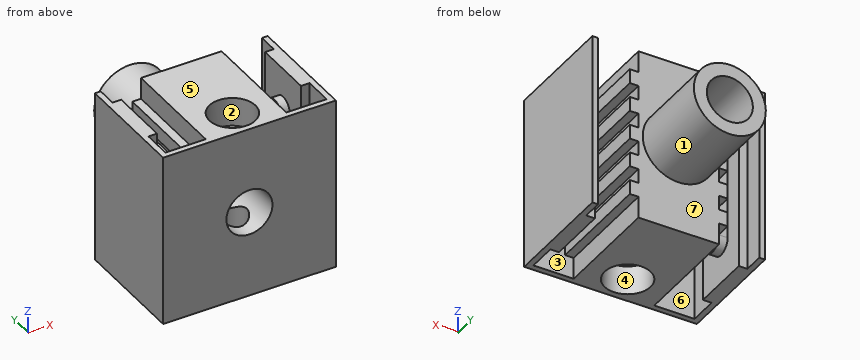
```python
from build123d import *

# Parameters (mm, degrees)
ESBO_O1_R                = 12.5
RESSALTO_EXTRUS_O1_DEPTH = 30
ESBO_O2_R                = 8
CORTE_EXTRUS_O1_DEPTH    = 15
ESBO_O3_W                = 3
ESBO_O3_H                = 5
CORTE_EXTRUS_O2_DEPTH    = 6.5
ESBO_O4_W                = 60
ESBO_O4_H                = 60
RESSALTO_EXTRUS_O2_DEPTH = 40
ESBO_O5_W                = 11
ESBO_O5_H                = 60
CORTE_EXTRUS_O3_DEPTH    = 35
ESBO_O6_W                = 11
ESBO_O6_H                = 60
CORTE_EXTRUS_O4_DEPTH    = 38
ESBO_O7_W                = 60
ESBO_O7_H                = 21
RESSALTO_EXTRUS_O3_DEPTH = 3.00002654
ESBO_O8_W                = 60
ESBO_O8_H                = 21
RESSALTO_EXTRUS_O4_DEPTH = 3.004451555
RESSALTO_EXTRUS_O5_DEPTH = 2.995218695
RESSALTO_EXTRUS_O6_START = 3
RESSALTO_EXTRUS_O6_DEPTH = 3
ESBO_O15_R               = 8
CORTE_EXTRUS_O5_DEPTH    = 70.462219947
ESBO_O19_W               = 5
ESBO_O19_H               = 38
ESBO_O19_W_2             = 7.5
CORTE_EXTRUS_O7_DEPTH    = 3
ESBO_O20_W               = 7.5
ESBO_O20_H               = 38
ESBO_O20_W_2             = 5
CORTE_EXTRUS_O8_DEPTH    = 3
ESBO_O21_R               = 8
CORTE_EXTRUS_O9_DEPTH    = 10
CORTE_EXTRUS_O10_START   = -10
ESBO_O22_R               = 8
CORTE_EXTRUS_O10_DEPTH   = 10
ESBO_O24_R               = 5
CORTE_EXTRUS_O11_DEPTH   = 71.710678119


with BuildPart() as part:
    # Esboço1 → Ressalto-extrusão1 (new body)
    with BuildSketch(Plane(origin=(0, 0, 0), x_dir=(1, 0, 0), z_dir=(0, 1, 0))):
        with Locations(Location((0, 0, 0), (0, 0, 270))):
            Circle(ESBO_O1_R)
    extrude(amount=RESSALTO_EXTRUS_O1_DEPTH)

    # Esboço2 → Corte-extrusão1 (cut)
    with BuildSketch(Plane(origin=(0, 30, 0), x_dir=(1, 0, 0), z_dir=(0, 1, 0))):
        with Locations(Location((0, 0, 0), (0, 0, 270))):
            Circle(ESBO_O2_R)
    extrude(amount=-CORTE_EXTRUS_O1_DEPTH, mode=Mode.SUBTRACT)

    # Esboço3 → Corte-extrusão2 (cut)
    with BuildSketch(Plane.XZ):
        Rectangle(ESBO_O3_W, ESBO_O3_H)
    extrude(amount=-CORTE_EXTRUS_O2_DEPTH, mode=Mode.SUBTRACT)

    # Esboço4 → Ressalto-extrusão2 (add)
    with BuildSketch(Plane.XZ):
        Rectangle(ESBO_O4_W, ESBO_O4_H)
    extrude(amount=RESSALTO_EXTRUS_O2_DEPTH)

    # Esboço5 → Corte-extrusão3 (cut)
    with BuildSketch(Plane(origin=(0, 0, 0), x_dir=(1, 0, 0), z_dir=(0, 1, 0))):
        with Locations((-22.5, 0)):
            Rectangle(ESBO_O5_W, ESBO_O5_H)
        with Locations((22.5, 0)):
            Rectangle(ESBO_O5_W, ESBO_O5_H)
    extrude(amount=-CORTE_EXTRUS_O3_DEPTH, mode=Mode.SUBTRACT)

    # Esboço6 → Corte-extrusão4 (cut)
    with BuildSketch(Plane(origin=(0, 0, 0), x_dir=(1, 0, 0), z_dir=(0, 1, 0))):
        with Locations((-22.5, 0)):
            Rectangle(ESBO_O6_W, ESBO_O6_H)
        with Locations((22.5, 0)):
            Rectangle(ESBO_O6_W, ESBO_O6_H)
    extrude(amount=-CORTE_EXTRUS_O4_DEPTH, mode=Mode.SUBTRACT)

    # Esboço7 → Ressalto-extrusão3 (add)
    with BuildSketch(Plane(origin=(-28, 0, 0), x_dir=(0, 0, -1), z_dir=(1, 0, 0))):
        with Locations((0, -17.5)):
            Rectangle(ESBO_O7_W, ESBO_O7_H)
    extrude(amount=RESSALTO_EXTRUS_O3_DEPTH)

    # Esboço8 → Ressalto-extrusão4 (add)
    with BuildSketch(Plane.ZY.offset(-28)):
        with Locations((0, -17.5)):
            Rectangle(ESBO_O8_W, ESBO_O8_H)
    extrude(amount=RESSALTO_EXTRUS_O4_DEPTH)

    # Esboço9 → Ressalto-extrusão5 (add)
    with BuildSketch(Plane.ZY.offset(-24.995548445)):
        with BuildLine():
            Line((-16, -13.5), (16, -13.5))
            ThreePointArc((16, -13.5), (20, -17.5), (16, -21.5))
            Line((16, -21.5), (-16, -21.5))
            ThreePointArc((-16, -21.5), (-20, -17.5), (-16, -13.5))
        make_face()
    extrude(amount=RESSALTO_EXTRUS_O5_DEPTH)

    # Esboço14 → Ressalto-extrusão6 (add)
    with BuildSketch(Plane(origin=(-24.99997346, 0, 0), x_dir=(0, 0, -1), z_dir=(1, 0, 0)).offset(RESSALTO_EXTRUS_O6_START)):
        with BuildLine():
            Line((-16, -13.5), (16, -13.5))
            ThreePointArc((16, -13.5), (20, -17.5), (16, -21.5))
            Line((16, -21.5), (-16, -21.5))
            ThreePointArc((-16, -21.5), (-20, -17.5), (-16, -13.5))
        make_face()
    extrude(amount=-RESSALTO_EXTRUS_O6_DEPTH)

    # Esboço15 → Corte-extrusão5 (cut, through all)
    with BuildSketch(Plane(origin=(0, 15, 0), x_dir=(1, 0, 0), z_dir=(0, 1, 0))):
        with Locations(Location((0, 0, 0), (0, 0, 270))):
            Circle(ESBO_O15_R)
    extrude(amount=-CORTE_EXTRUS_O5_DEPTH, mode=Mode.SUBTRACT)

    # Esboço19 → Corte-extrusão7 (cut)
    with BuildSketch(Plane.ZY.offset(17)):
        with Locations((-15, -19)):
            Rectangle(ESBO_O19_W, ESBO_O19_H)
        with Locations((-26.25, -19)):
            Rectangle(ESBO_O19_W_2, ESBO_O19_H)
        with Locations((-5, -19)):
            Rectangle(ESBO_O19_W, ESBO_O19_H)
        with Locations((5, -19)):
            Rectangle(ESBO_O19_W, ESBO_O19_H)
        with Locations((15, -19)):
            Rectangle(ESBO_O19_W, ESBO_O19_H)
        with Locations((26.25, -19)):
            Rectangle(ESBO_O19_W_2, ESBO_O19_H)
    extrude(amount=-CORTE_EXTRUS_O7_DEPTH, mode=Mode.SUBTRACT)

    # Esboço20 → Corte-extrusão8 (cut)
    with BuildSketch(Plane(origin=(17, 0, 0), x_dir=(0, 0, -1), z_dir=(1, 0, 0))):
        with Locations((-26.25, -19)):
            Rectangle(ESBO_O20_W, ESBO_O20_H)
        with Locations((-15, -19)):
            Rectangle(ESBO_O20_W_2, ESBO_O20_H)
        with Locations((-5, -19)):
            Rectangle(ESBO_O20_W_2, ESBO_O20_H)
        with Locations((5, -19)):
            Rectangle(ESBO_O20_W_2, ESBO_O20_H)
        with Locations((15, -19)):
            Rectangle(ESBO_O20_W_2, ESBO_O20_H)
        with Locations((26.25, -19)):
            Rectangle(ESBO_O20_W, ESBO_O20_H)
    extrude(amount=-CORTE_EXTRUS_O8_DEPTH, mode=Mode.SUBTRACT)

    # Esboço21 → Corte-extrusão9 (cut)
    with BuildSketch(Plane.XY.offset(30)):
        with Locations((0, -30)):
            Circle(ESBO_O21_R)
    extrude(amount=-CORTE_EXTRUS_O9_DEPTH, mode=Mode.SUBTRACT)

    # Esboço22 → Corte-extrusão10 (cut)
    with BuildSketch(Plane(origin=(0, 0, -30), x_dir=(-1, 0, 0), z_dir=(0, 0, -1)).offset(CORTE_EXTRUS_O10_START)):
        with Locations(Location((0, -30, 0), (0, 0, 180))):
            Circle(ESBO_O22_R)
    extrude(amount=CORTE_EXTRUS_O10_DEPTH, mode=Mode.SUBTRACT)

    # Esboço24 → Corte-extrusão11 (cut, through all)
    with BuildSketch(Plane(origin=(0, 0, -20), x_dir=(-1, 0, 0), z_dir=(0, 0, -1))):
        with Locations(Location((0, -30, 0), (0, 0, 270))):
            Circle(ESBO_O24_R)
    extrude(amount=-CORTE_EXTRUS_O11_DEPTH, mode=Mode.SUBTRACT)


solid = part.part
```
Part model, mm, in its own coordinate system. Face numbers are marked on the shaded views. A direction names the side the tool comes from. Round coordinates to 2 decimals unless told otherwise and drop trailing zeros. Loops run counter-clockwise (first coordinate to the right, second up) from the corner with the lowest first, then second, coordinate; pieces in that order, holes last.
Item 1: Cut at A-A, the plane x = 0. Give the cut face in (y, z), then the cut area to 3 significant figures.
Item 2: Cut at B-B, the plane y = -17.5. State how many separate pieces and enclosed holes the cut face has, then the cut area to 3 significant figures.
Item 3: Drop flat-ended pins along their axis: P1, Ø0.9, axis at x = -15, y = -27.5, coming from the -Z side; P2, Ø1, axis at x = -2, y = -25.5, coming from the +Z side; P3, Ø6, axis at x = -14, y = 12, coming from the +Z side. Give the stop position or say it passes through.
Item 4: 3-axis set-ups, long thin cutter, end or side, ignore diameter. For the marked faces 1, 2, 3 and 4: which of +Z, -Z, +X, -X, +Y, -Y reach the whole face in a straight line?
Item 5: Drill centre lines: line 1 (X direction, y = -5, z = -20.5); line 2 (X direction, y = -21, z = -27); line 3 (Y direction, x = 22.5, z = 5). Where is each one in solid material? Low to high.
Item 6: Mould opens along Y. For the marked faces 5, 6 and 7 say: +Y half, -Y half, draft (parallel to the pull), parting line (faces both ways), or undercut.
Item 7: Cut at D-D, the plane x = 10. Give the cut face in (y, z), then the cut area to 3 significant figures.
A:
1. outline: (-40, -30) - (-38, -30) - (-38, -20) - (-35, -20) - (-35, -8) - (-40, -8) - close; (-40, 8) - (-35, 8) - (-35, 20) - (-38, 20) - (-38, 30) - (-40, 30) - close; (-25, -20) - (-22, -20) - (-22, -30) - (0, -30) - (0, -12.5) - (30, -12.5) - (30, -8) - (-25, -8) - close; (-25, 8) - (30, 8) - (30, 12.5) - (0, 12.5) - (0, 30) - (-22, 30) - (-22, 20) - (-25, 20) - close
1. area: 1,470 mm2
2. separate pieces: 3
2. enclosed holes: 1
2. area: 2,470 mm2
3. P1: stops at z = -22.5
3. P2: stops at z = 20
3. P3: stops at z = 5.94
4. face 1: +Y
4. face 2: +Z
4. face 3: none
4. face 4: -Z
5. line 1: x = -30 to -28, -17 to 17, 28 to 30
5. line 2: x = -30 to -25, -14 to 14, 25 to 30
5. line 3: y = -40 to -38, -21.5 to -13.5
6. face 5: draft
6. face 6: undercut
6. face 7: +Y half
7. outline: (-40, -30) - (0, -30) - (0, -7.5) - (30, -7.5) - (30, 7.5) - (0, 7.5) - (0, 30) - (-40, 30) - close
7. area: 2,850 mm2
